Here's the drawing with two shaded views (mm, measured from the low corner). I have some questions. A direction names the side the tool comes from. Round coordinates to 2 decimals unless told otherwise and drop trailing zeros. Loops run counter-clockwise (first coordinate to the right, second up) from the corner with the lowest first, then second, coordinate; pieces in that order, holes last. Notation, with made-up numbers: M 79,-2 L 115,-2 A7 cw 115,2 Z; hole C 85,2 d11. An arc over 180 degrees is marked long. One line per item, written item: value. Start each with the question number.
Q1. Imagine slicing it at A-A (z = 18). Please give me the cut outline in (x, y), then the cut area to 3 significant figures.
Q2. Imagine slicing it at B-B (y = 24). Please give me the cut outline in (x, z).
Q3. Please list where these lines run through material, in increasing order: line 1 along Y through (x, z) = (6, 16); line 2 along Z through (x, y) = (28.5, 20); line 3 along Y through (x, z) = (20, 2.8).
Q4. Imagine slicing it at C-C (x = 100). Please give me the cut outline in (y, z).
Q5. Imagine slicing it at D-D (x = 87.5). Please give me the cut outline in (y, z).
Q6. Thinking about a two-plate mould opening in Y: for the marked faces 3, 4 and 5, which applies, released by +Y, released by -Y, zero draft, split by the parting line, or undercut?
Q7. Which directions (+Z, -Z, +X, -X, +Y, -Y) give clear straight access to the entire face, cutting with the end or side of a thin tool? Please do the marked faces 1 and 2.
Q8. I'm going to push flat-ended pins straight in: pin 1 Ø8 at (y, z) = (38, 16.5) entering from +X; pin 2 Ø1 at (x, z) = (43.5, 14) entering from -Y; pin 3 Ø7 at (x, y) = (20, 24) entering from +Z. Where does each tip first touch, or does it pass through?
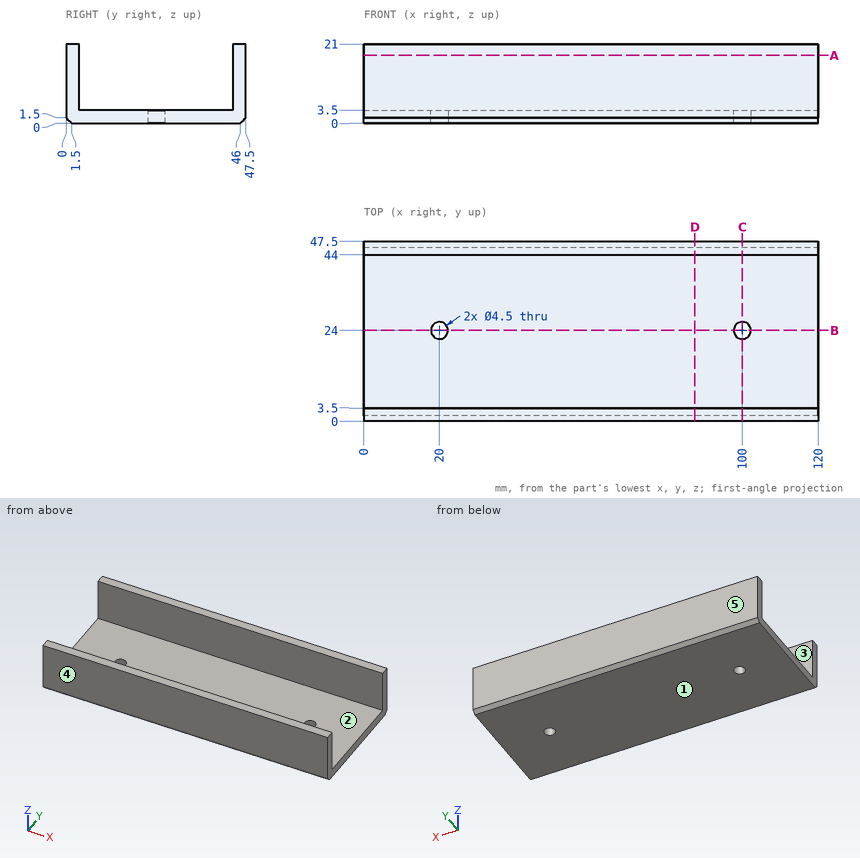
Report:
1. outline: M 0,0 L 120,0 L 120,3.5 L 0,3.5 Z; M 0,44 L 120,44 L 120,47.5 L 0,47.5 Z
1. area: 840 mm²
2. outline: M 0,0 L 17.75,0 L 17.75,3.5 L 0,3.5 Z; M 22.25,0 L 97.75,0 L 97.75,3.5 L 22.25,3.5 Z; M 102.25,0 L 120,0 L 120,3.5 L 102.25,3.5 Z
3. line 1: y = 0 to 3.5, 44 to 47.5
3. line 2: z = 0 to 3.5
3. line 3: y = 0 to 21.75, 26.25 to 47.5
4. outline: M 0,1.5 L 1.5,0 L 21.75,0 L 21.75,3.5 L 3.5,3.5 L 3.5,21 L 0,21 Z; M 26.25,0 L 46,0 L 47.5,1.5 L 47.5,21 L 44,21 L 44,3.5 L 26.25,3.5 Z
5. outline: M 0,1.5 L 1.5,0 L 46,0 L 47.5,1.5 L 47.5,21 L 44,21 L 44,3.5 L 3.5,3.5 L 3.5,21 L 0,21 Z
6. face 3: undercut
6. face 4: released by -Y
6. face 5: released by +Y
7. face 1: -Z, +X, -X, +Y, -Y
7. face 2: +Z, +X, -X
8. pin 1: passes through
8. pin 2: stops at y = 0
8. pin 3: stops at z = 3.5
